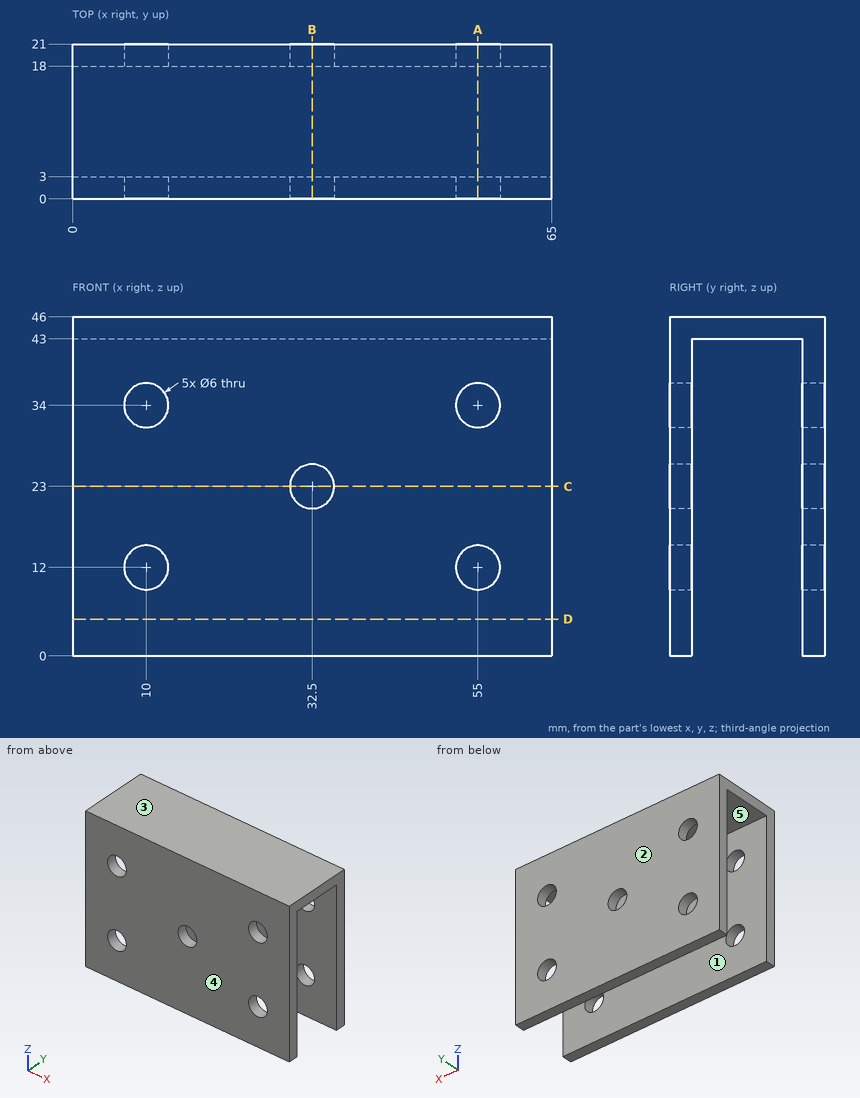
Job drawing, mm, ordinate dimensions from the low corner. One solid piece. A direction names the side the tool comes from. Coordinates: 2 decimals unless noted, no trailing zeros. Order: outer loops, then holes, each group sorted by start corner. A loop starts at its lowest first (then second) coordinate and runs counter-clockwise, first axis right, second up. Notation, with made-up numbers: (43.5, 54) - (100.5, 54) arc R12 cw to (100.5, 74) - close; hole circle Ø11 at (75, 12). An arc over 180 degrees is marked (long way). Write each question's results on one line, items separated by ' | '. Start each with the question number.
Item 1: Band-saw the part on A-A on x = 55. Write the cut outline in (y, z).
Item 2: Band-saw the part on B-B on x = 32.5. Write the cut outline in (y, z).
Item 3: Wall check: probe 1 along X at (y, z) = (19, 34); probe 2 along Y at (x, z) = (37, 18); probe 3 along Z at (x, y) = (8, 18.5). Give the ranges that are in metal, low to high. Write a range as [from, to].
Item 4: Flat gauge pins, fed straight in: pin 1 (8 mm diameter, centred on x = 55, z = 12, fed in from -Y); pin 2 (1.5 mm diameter, centred on y = 4.5, z = 25.5, fed in from +X); pin 3 (7.5 mm diameter, centred on x = 27.5, y = 12, fed in from -Z). Where does each tip first touch, or does it go through?
Item 5: Band-saw the part on D-D on z = 5. Write the cut outline in (x, y).
Item 6: Tool access for the marked faces 1 and 2: list every direction of +Z, -Z, +X, -X, +Y, -Y with a clear straight run to the whole face (end or side of a thin tool).
Item 7: Mould opens along Y. For the marked faces 3, 4 and 5 say: released by +Y, released by -Y, zero draft, split by the parting line, or undercut.
Item 8: Band-saw the part on C-C on z = 23. Write the cut outline in (x, y).
Numbers:
1) outline: (0, 0) - (3, 0) - (3, 9) - (0, 9) - close; (0, 15) - (3, 15) - (3, 31) - (0, 31) - close; (0, 37) - (3, 37) - (3, 43) - (18, 43) - (18, 37) - (21, 37) - (21, 46) - (0, 46) - close; (18, 0) - (21, 0) - (21, 9) - (18, 9) - close; (18, 15) - (21, 15) - (21, 31) - (18, 31) - close
2) outline: (0, 0) - (3, 0) - (3, 20) - (0, 20) - close; (0, 26) - (3, 26) - (3, 43) - (18, 43) - (18, 26) - (21, 26) - (21, 46) - (0, 46) - close; (18, 0) - (21, 0) - (21, 20) - (18, 20) - close
3) probe 1: [0, 7], [13, 52], [58, 65] | probe 2: [0, 3], [18, 21] | probe 3: [0, 9.76], [14.24, 31.76], [36.24, 46]
4) pin 1: y = 0 | pin 2: through | pin 3: z = 43
5) outline: (0, 0) - (65, 0) - (65, 3) - (0, 3) - close; (0, 18) - (65, 18) - (65, 21) - (0, 21) - close
6) face 1: -Z, +X, -X | face 2: +Z, -Z, +X, -X, +Y
7) face 3: zero draft | face 4: released by -Y | face 5: undercut
8) outline: (0, 0) - (29.5, 0) - (29.5, 3) - (0, 3) - close; (0, 18) - (29.5, 18) - (29.5, 21) - (0, 21) - close; (35.5, 0) - (65, 0) - (65, 3) - (35.5, 3) - close; (35.5, 18) - (65, 18) - (65, 21) - (35.5, 21) - close
